Work out the finished part from the listing and answer in its coordinate system (mm). A direction names the side the tool comes from. Round coordinates to 2 decimals unless told otherwise and drop trailing zeros. Write each loop counter-clockwise with the first axis right and the second up, starting at its lowest first coordinate (ties: lowest second). Pieces come first, ordered by that corner, then holes. Notation, with made-up numbers: (-38, 36) - (13, 36) arc R35 cw to (13, 69) - close; hole circle Ø8 at (86.25, 68). An arc over 180 degrees is marked (long way). Answer as a JSON object with one key per item and string values.
```python
from build123d import *

# Parameters (mm, degrees)
F0_W     = 93.204498291
F0_H     = 98.337136209
F1_DEPTH = 25.4
F2_DEPTH = 45
F4_D     = 6.35
F7_T     = -10
F8_W     = 36.6022491455
F8_H     = 17.213357389
F9_DEPTH = 25.4


# Not quite as in the source:
# - the program builds the solid bodies; features that only make, move or delete a surface that nothing else refers to are left out


with BuildPart() as f1:
    # F0 (on Top) → F1 (new body)
    with BuildSketch(Plane.XY):
        with Locations((-3.3413916826, 1.5083067119)):
            Rectangle(F0_W, F0_H)
    extrude(amount=F1_DEPTH)

    # F2 (add): a face of the model
    f2_faces = [f1.faces().sort_by_distance(p)[0] for p in [
        (-3.3413916826, 1.5083067119, 25.4),
    ]]
    extrude(f2_faces, amount=F2_DEPTH)

    # F4 (through all)
    with Locations(Plane.XY.offset(70.4)):
        with Locations((0, 0)):
            Hole(F4_D / 2)

    # F7
    f7_openings = [f1.faces().sort_by_distance(p)[0] for p in [
        (-3.352977, 1.513536, 70.4),
    ]]
    offset(amount=F7_T, openings=f7_openings)

    # F8 (on face) → F9 (join)
    with BuildSketch(Plane.XY.offset(10)):
        with Locations((-21.6425162554, 32.0701961219)):
            Rectangle(F8_W, F8_H)
    extrude(amount=F9_DEPTH)


solid = f1.part
```
Item 1: A cutting plane is placed at D-D (y = 0). Write down the section's boundary in (x, z) (3 decimals), and give its area (3 significant figures).
Results found:
{"outline": "(-49.944, 0) - (-3.175, 0) - (-3.175, 70.4) - (-13.175, 70.4) - (-13.175, 10) - (-39.944, 10) - (-39.944, 70.4) - (-49.944, 70.4) - close; (3.175, 0) - (43.261, 0) - (43.261, 70.4) - (33.261, 70.4) - (33.261, 10) - (13.175, 10) - (13.175, 70.4) - (3.175, 70.4) - close", "area": "3,280 mm²"}
Item 2: A cutting plane is placed at C-C (y = -28.5). Write down the section's boundary in (x, z), and give its area (3 significant figures).
Results found:
{"outline": "(-49.94, 0) - (43.26, 0) - (43.26, 70.4) - (33.26, 70.4) - (33.26, 10) - (-39.94, 10) - (-39.94, 70.4) - (-49.94, 70.4) - close", "area": "2,140 mm²"}
Item 3: A cutting plane is placed at A-A (x = 0). Write down the section's boundary in (y, z) (3 decimals), and give its area (3 significant figures).
Results found:
{"outline": "(-47.66, 0) - (-3.175, 0) - (-3.175, 70.4) - (-13.175, 70.4) - (-13.175, 10) - (-37.66, 10) - (-37.66, 70.4) - (-47.66, 70.4) - close; (3.175, 0) - (50.677, 0) - (50.677, 70.4) - (40.677, 70.4) - (40.677, 10) - (13.175, 10) - (13.175, 70.4) - (3.175, 70.4) - close", "area": "3,340 mm²"}
Item 4: For faces 4 (the cylindrical face through (2.86, -12.86, 39.78)), 5 (the flat face through (-4, 2, 0)), determine the directions among +Z, -Z, +X, -X, +Y, -Y from which every point of the face is accessible in a straight line to the end or side of a thin tool.
Results found:
{"face 4": "+Z", "face 5": "-Z, +X, -X, +Y, -Y"}
Item 5: Determine the mould class of faces 1 (the flat face through (43.261, 1, 35)), 2 (the flat face through (-4, 50.677, 35)), 3 (the flat face through (-39.944, 1, 40)) for opening direction Y: pulls with the +Y half, pulls with the -Y half, needs draft (parallel to the pull), parting line crosses it, or undercut.
Results found:
{"face 1": "needs draft", "face 2": "pulls with the +Y half", "face 3": "undercut"}
Item 6: A cutting plane is placed at B-B (z = 32.5). Write down the section's boundary in (x, y) (3 decimals), and give its area (3 significant figures).
Results found:
{"outline": "(-49.944, -47.66) - (43.261, -47.66) - (43.261, 50.677) - (-49.944, 50.677) - close; circle Ø26.35 at (0, 0); hole (-39.944, -37.66) - (33.261, -37.66) - (33.261, 40.677) - (-3.341, 40.677) - (-3.341, 23.464) - (-39.944, 23.464) - close; hole circle Ø6.35 at (0, 0)", "area": "4,570 mm²"}
Item 7: Consider line 1 along Y through (x, z) = (0, 39) (3 decimals); line 2 along Y through (x, z) = (-19, 38); line 3 along X through (y, z) = (-36.5, 22). Determine where each line is inside the solid, lowest interval first.
Results found:
{"line 1": "-47.66 to -37.66, -13.175 to -3.175, 3.175 to 13.175, 40.677 to 50.677", "line 2": "-47.66 to -37.66, 40.68 to 50.68", "line 3": "-49.94 to -39.94, 33.26 to 43.26"}
Item 8: Each of these flat-tipped pins is pushed along its axis until it touches: P1, Ø4, axis at x = 8.5, y = 36.5, coming from the +Z side; P2, Ø1, axis at x = -23.5, y = 18.5, coming from the -Z side; P3, Ø8.5, axis at x = -30.5, y = 35.5, coming from the +Z side. Where does it stop, or does it pass through?
Results found:
{"P1": "z = 10", "P2": "z = 0", "P3": "z = 35.4"}
